Could you check a few things on this drawing? It's one solid part, dimensions in mm from its lowest x, y, z. Coordinates: 2 decimals unless noted, no trailing zeros. Loops run counter-clockwise (first coordinate to the right, second up) from the corner with the lowest first, then second, coordinate; pieces in that order, holes last. Notation, with made-up numbers: M 41.5,-23.5 L 58.5,-23.5 A17 cw 58.5,-9.5 Z; hole C -27.75,78 d8. An arc over 180 degrees is marked long. Answer as a JSON object with one key per item and string values. Group by question number.
Item 1: If I drill on line 1 (Z direction, x = 447.5, y = 11.5); line 2 (X direction, y = 3, z = 219), over which ranges is the centre line in solid material (lowest first)?
Item 2: Suppose I cut it at A-A (y = 8). Write out the boundary of the cut face in (x, z).
Item 3: Suppose I cut it at C-C (z = 444). Write out the boundary of the cut face in (x, y).
Item 4: Suppose I cut it at B-B (x = 426.5). Write out the boundary of the cut face in (y, z), then the cut area to 3 significant figures.
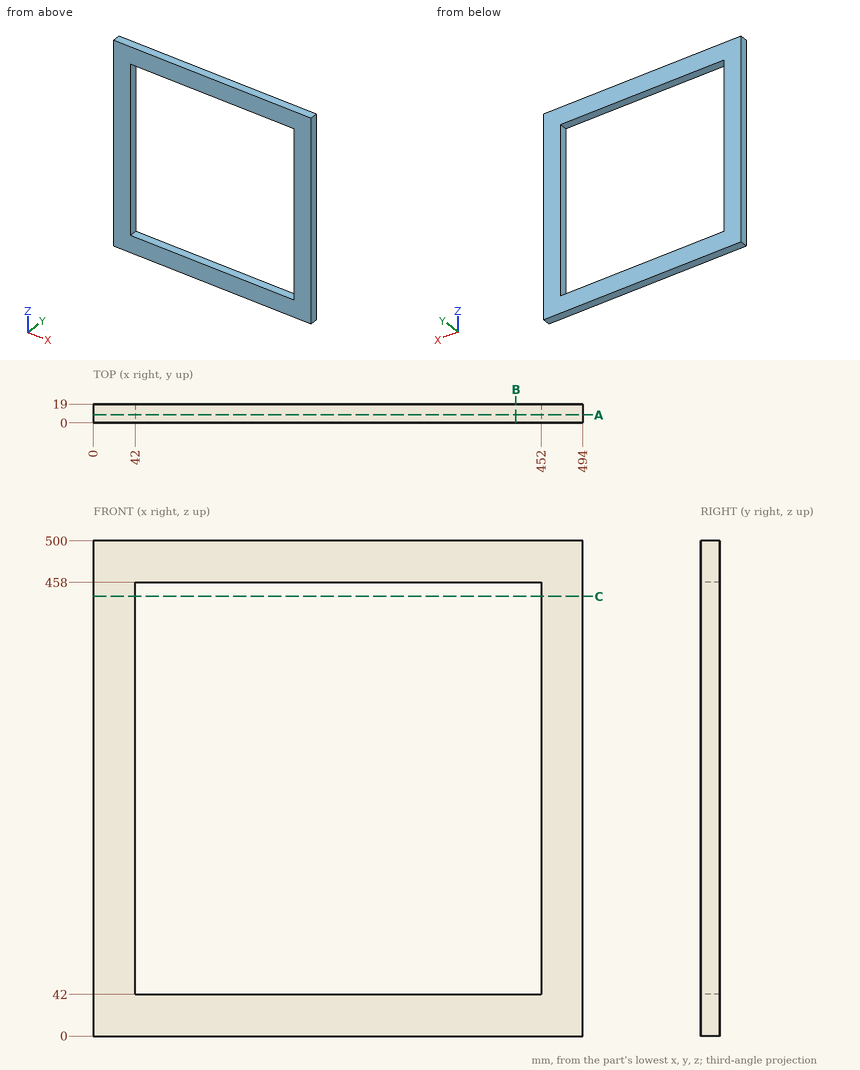
From the geometry:
{
 "1": {"line 1": "0 to 42, 458 to 500", "line 2": "0 to 42, 452 to 494"},
 "2": {"outline": "M 0,0 L 494,0 L 494,500 L 0,500 Z; hole M 42,42 L 452,42 L 452,458 L 42,458 Z"},
 "3": {"outline": "M 0,0 L 42,0 L 42,19 L 0,19 Z; M 452,0 L 494,0 L 494,19 L 452,19 Z"},
 "4": {"outline": "M 0,0 L 19,0 L 19,42 L 0,42 Z; M 0,458 L 19,458 L 19,500 L 0,500 Z", "area": "1,600 mm2"}
}
